Answer from the drawing. Dimensions are ordinates in mm from the lowest x, y and z of the part. A direction names the side the tool comes from. Give positions to 0.01 mm unless a question says otherwise; leave off trailing zeros. Loops run counter-clockwise (first coordinate to the right, second up) from the corner with the lowest first, then second, coordinate; pieces in that order, holes last.
Item 1: Section A-A, the plane x = 7.25 is taken. Give the vertices of the cut face in (y, z), and give its area (3 significant figures).
Item 2: Section B-B, the plane z = 8.25 is taken. Give the vertices of the cut face in (x, y), and give its area (3 significant figures).
Item 3: Each of these flat-tipped pins is pushed along its axis until it touches: pin 1 Ø0.9 at (x, y) = (9, 25) entering from +Z; pin 2 Ø3 at (x, y) = (33.25, 7) entering from -Z; pin 3 Ø3 at (x, z) = (3.3, 3) entering from +Y; pin 4 Ø2.5 at (x, z) = (24, 7.5) entering from +Y. Where does it stop, or does it pass through?
Item 4: Section C-C, the plane y = 7 is taken. Give the vertices of the cut face in (x, z).
Item 5: Consider line 1 along Y through (x, z) = (7.25, 2.3); line 2 along Z through (x, y) = (12.3, 1.3) (3 decimals); line 3 along X through (y, z) = (1.5, 4). Determine where each line is inside the solid, lowest interval first.
Item 6: Section D-D, the plane z = 5.25 is taken. Give the vertices of the cut face in (x, y).
Item 7: A tool of negligible diameter and unlimited length cuts with its end or side. For the marked faces 1, 2, 3, 4 and 5, from which of +Z, -Z, +X, -X, +Y, -Y can it reach the whole face along a straight path? Write none if from no direction.
Item 8: The mould has two halves that part along X. Classify the marked faces 6, 7, 8 and 9: pulls with the +X half, pulls with the -X half, needs draft (parallel to the pull), parting line crosses it, or undercut.
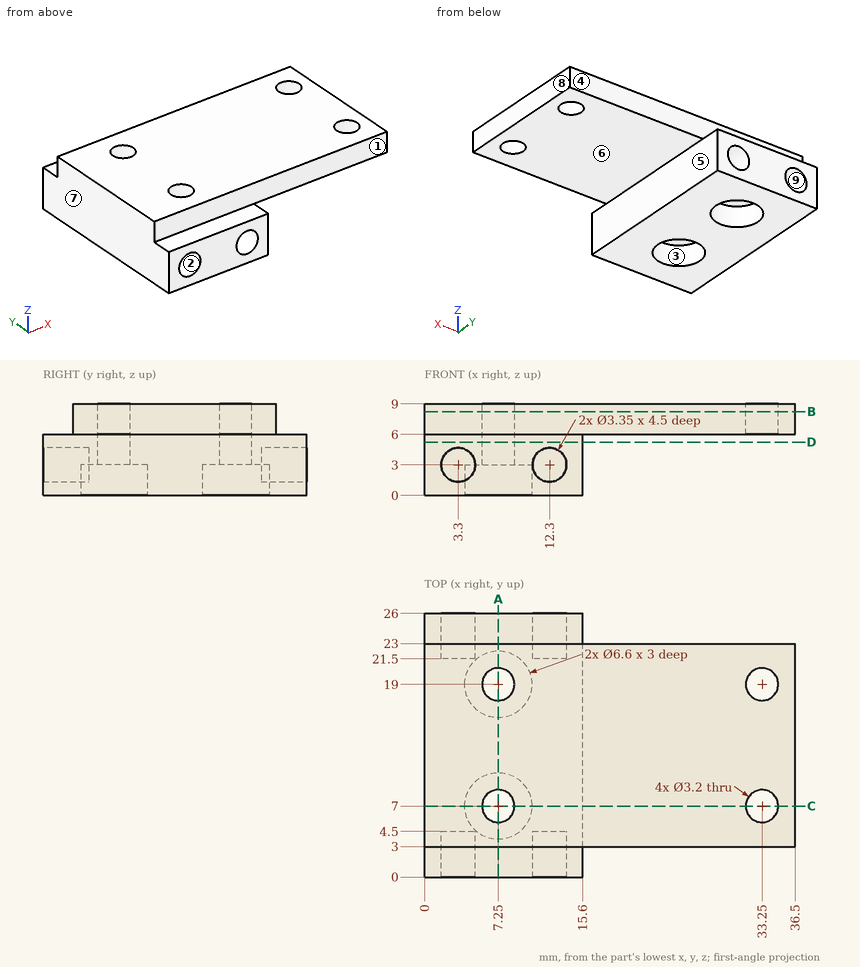
Worked answers:
1. outline: (0, 0) - (3.7, 0) - (3.7, 3) - (5.4, 3) - (5.4, 9) - (3, 9) - (3, 6) - (0, 6) - close; (8.6, 3) - (10.3, 3) - (10.3, 0) - (15.7, 0) - (15.7, 3) - (17.4, 3) - (17.4, 9) - (8.6, 9) - close; (20.6, 3) - (22.3, 3) - (22.3, 0) - (26, 0) - (26, 6) - (23, 6) - (23, 9) - (20.6, 9) - close
1. area: 138 mm2
2. outline: (0, 3) - (36.5, 3) - (36.5, 23) - (0, 23) - close; hole circle Ø3.2 at (7.25, 7); hole circle Ø3.2 at (7.25, 19); hole circle Ø3.2 at (33.25, 7); hole circle Ø3.2 at (33.25, 19)
2. area: 698 mm2
3. pin 1: stops at z = 6
3. pin 2: passes through
3. pin 3: stops at y = 21.5
3. pin 4: stops at y = 23
4. outline: (0, 0) - (3.95, 0) - (3.95, 3) - (5.65, 3) - (5.65, 9) - (0, 9) - close; (8.85, 3) - (10.55, 3) - (10.55, 0) - (15.6, 0) - (15.6, 6) - (31.65, 6) - (31.65, 9) - (8.85, 9) - close; (34.85, 6) - (36.5, 6) - (36.5, 9) - (34.85, 9) - close
5. line 1: y = 0 to 3.7, 10.3 to 15.7, 22.3 to 26
5. line 2: z = 0 to 1.325, 4.675 to 6
5. line 3: x = 0 to 1.96, 4.64 to 10.96, 13.64 to 15.6
6. outline: (0, 0) - (15.6, 0) - (15.6, 26) - (0, 26) - close; hole circle Ø3.2 at (7.25, 7); hole circle Ø3.2 at (7.25, 19)
7. face 1: +Z, +X, -X, -Y
7. face 2: -Y
7. face 3: -Z
7. face 4: +Z, +X, -X, +Y
7. face 5: -Z, +X, +Y, -Y
8. face 6: needs draft
8. face 7: pulls with the -X half
8. face 8: pulls with the +X half
8. face 9: undercut
